Geometry: see drawing. Coordinates: mm, zero at the bounding-box minimum. A direction names the side the tool comes from. Give positions to 0.01 mm unless a question says otherwise; leave off trailing zeros. Write each loop counter-clockwise with the first axis right and the second up, starting at its lowest first coordinate (ties: lowest second). Pieces come first, ordered by that corner, then holes. Notation, with made-up numbers: M 32.25,31 L 75.25,31 A26 cw 75.25,69 Z; hole C 36.25,-34 d7. An arc over 180 degrees is marked long. Use a Markdown table: item, result. Add a question column.
(1) Cut plane D-D (y = 4.5). Output: boundary loops of the cut face in (x, z), plus the area to 3 significant figures.
(2) Cut plane A-A (z = 18.5). Output: boundary loops of the cut face in (x, y), plus the area to 3 significant figures.
(3) Pin query (flat end, axial travel): pin 1 Ø4 at (x, z) = (15, 21) entering from +Y; pin 2 Ø1.5 at (y, z) = (27.5, 5) entering from +X; pin 3 Ø4 at (y, z) = (26, 25) entering from -X; pin 4 Ø3.5 at (y, z) = (18.5, 18.5) entering from -X. Return the tip coordinate at first contact, or that it passes through.
(4) Draft query along Z for the marked faces 1, 2 and 3. Return one class per face: released by +Z, released by -Z, zero draft, split by the parting line, or undercut.
(5) Reachability of the marked faces 4, 5 and 6 from +Z, -Z, +X, -X, +Y, -Y: full face, straight path, thin tool, end or side. Return the list, or none.
(6) Cut plane C-C (x = 4.25). Output: boundary loops of the cut face in (y, z).
(7) Material intervals for L1, parallel to Y at x = 23, z = 18.5; L2, parallel to Y at x = 24.6, z = 18.5; L3, parallel to Z at x = 8, y = 6, sorted ascending.
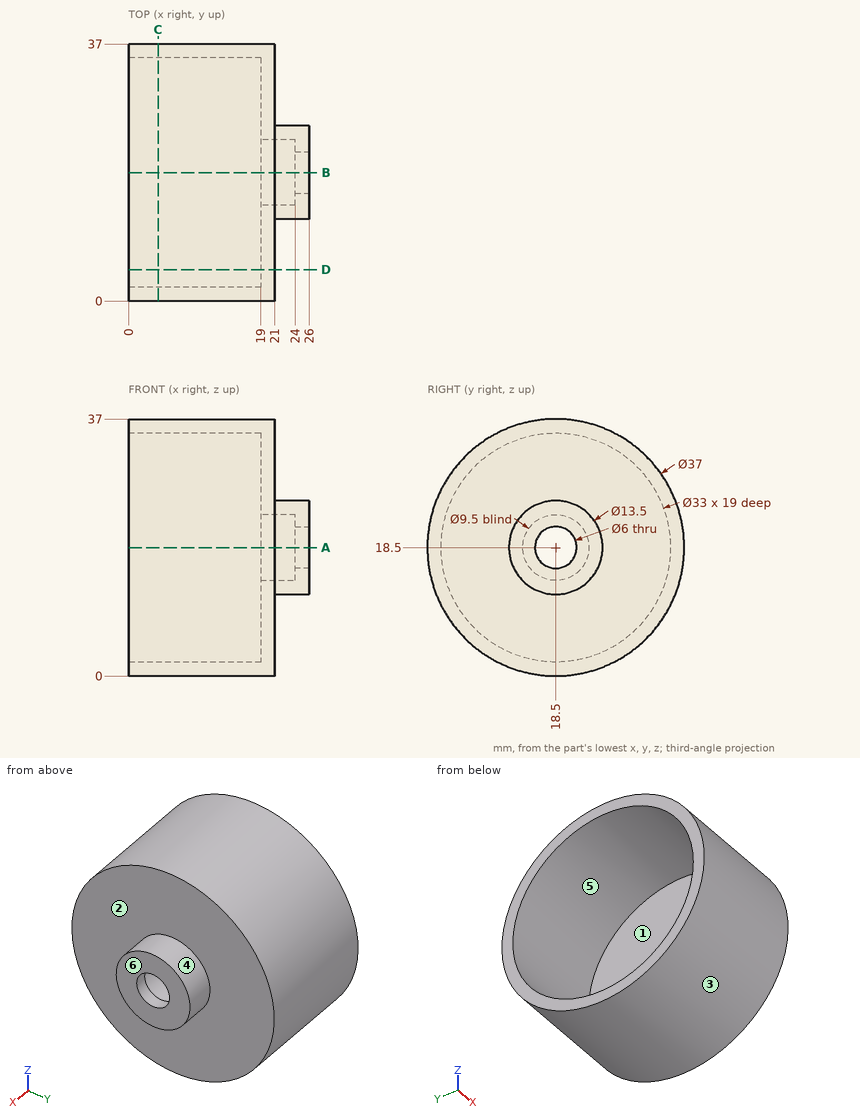
Answer list:
| question | item | result |
|---|---|---|
| 1 | outline | M 0,6.41 L 21,6.41 L 21,30.59 L 0,30.59 L 0,27.23 L 19,27.23 L 19,9.77 L 0,9.77 Z |
| 1 | area | 176 mm² |
| 2 | outline | M 0,0 L 21,0 L 21,11.75 L 26,11.75 L 26,15.5 L 24,15.5 L 24,13.75 L 19,13.75 L 19,2 L 0,2 Z; M 0,35 L 19,35 L 19,23.25 L 24,23.25 L 24,21.5 L 26,21.5 L 26,25.25 L 21,25.25 L 21,37 L 0,37 Z |
| 2 | area | 158 mm² |
| 3 | pin 1 | y = 36.99 |
| 3 | pin 2 | x = 21 |
| 3 | pin 3 | x = 19 |
| 3 | pin 4 | through |
| 4 | face 1 | undercut |
| 4 | face 2 | zero draft |
| 4 | face 3 | split by the parting line |
| 5 | face 4 | +X |
| 5 | face 5 | -X |
| 5 | face 6 | +Z, -Z, +X, +Y, -Y |
| 6 | outline | C 18.5,18.5 d37; hole C 18.5,18.5 d33 |
| 7 | L1 | 11.75 to 13.75, 23.25 to 25.25 |
| 7 | L2 | 11.75 to 15.5, 21.5 to 25.25 |
| 7 | L3 | 4.86 to 7.73, 29.27 to 32.14 |
